Source: CAD feature listing. Evaluate the final solid. Frame: model axes, mm. A direction names the side the tool comes from. Give positions to 0.01 mm unless a question says otherwise; leave off trailing zeros. Loops run counter-clockwise (first coordinate to the right, second up) from the corner with the lowest first, then second, coordinate; pieces in that order, holes last. Notation, with made-up numbers: (82.5, 72.5) - (87.5, 72.5) arc R18 cw to (87.5, 77.5) - close; hole circle Ø8 at (3, 24.5). An arc over 180 degrees is marked (long way). Write each question's results on one line, items separated by ' | '. Start each with the question number.
(1) Reachability of faces 1 (the flat face through (4, -29, -7)), 2 (the flat face through (0, 29, 0)) from +Z, -Z, +X, -X, +Y, -Y: full face, straight path, thin tool, end or side. Return the list, or none.
(2) Material intervals for line 1 along X through (y, z) = (21.5, 0.25); line 2 along Y through (x, z) = (2.5, -8.75), sorted ascending. Write a range as [from, to].
(3) Contact query for flat-ended pins moving along their axis: pin 1 (1.5 mm diameter, centred on x = 2, y = 8.5, fed in from -Z); pin 2 (4 mm diameter, centred on y = 21, z = -3.5, fed in from +X); pin 3 (8 mm diameter, centred on y = -18, z = 7.5, fed in from +X). Output: stop coordinate, or through.
(4) Cut plane C-C on y = -2.5. Return the cut outline in (x, z), then the cut area to 3 significant figures.
Autodesk Fusion 360 part; units mm, degrees
sketch "Sketch1" plane through (0, 0, 0) normal (0, 1, 0) x (1, 0, 0)
  circle A0 centre (0, 0) radius 7.5
  circle A1 centre (0, 0) radius 12
  dimension "d1" = 15
  dimension "d2" = 24
extrude "Extrude1" add sketch "Sketch1" along normal mid plane 58 contours A0 makes body 1
extrude "Extrude2" add sketch "Sketch1" along normal blind 0 and the other way blind 4 from surface at -29 contours A0 | A1 bodies 1
fillet "Fillet1" radius 2 2 edges at (-11.1879, -33, -4.3394) (-11.1879, -29, 4.3394) on bodies 1
copy_body "Body->Comp1" bodies 1 removing the originals makes body 2 in component "Component"
fillet "Fillet1'" radius 1.5 1 edges at (-6.9925, 29, 2.7121) on bodies 2 in component "Component"
component "Component" placed x (1, 0, 0) y (0, 1, 0) z (0, 0, 1) at (0, 0, 0)
Ans:
1) face 1: +Y | face 2: +Z, -Z, +X, -X, +Y
2) line 1: [-7.5, 7.5] | line 2: [-33, -29]
3) pin 1: z = -7.4 | pin 2: x = 7.35 | pin 3: x = 6.63
4) outline: circle Ø15 at (0, 0) | area: 177 mm^2
